The listing builds one solid part. Answer for the finished solid, in the listing's coordinates (mm). A direction names the side the tool comes from. Give positions to 0.01 mm unless a question says otherwise; leave off trailing zeros. Order: outer loops, then holes, each group sorted by start corner. A loop starts at its lowest first (then second) coordinate and runs counter-clockwise, first axis right, second up. Notation, with made-up numbers: (51.25, 13.25) -> (107.25, 13.25) arc R19 ccw to (107.25, 28.25) -> close; hole circle Ø8 at (-16, 34.5). An arc over 180 degrees is marked (long way). One line per question, with ' | ' between items. Start each with the question number.
```python
from build123d import *

# Parameters (mm, degrees)
F0_W     = 463.55
F0_H     = 158.75
F1_DEPTH = 457.2
F3_DEPTH = 158.751
F4_W     = 44.45
F4_H     = 304.8
F5_DEPTH = 381.001


with BuildPart() as f1:
    # F0 (on Top) → F1 (new body)
    with BuildSketch(Plane.XY):
        Rectangle(F0_W, F0_H)
    extrude(amount=F1_DEPTH)

    # F2 (on face) → F3 (cut, through all)
    with BuildSketch(Plane.XZ.offset(79.375)):
        Polygon((-149.225, 0), (-149.225, 304.8), (-231.775, 381), (-231.775, 0), align=None)
        Polygon((149.225, 304.8), (149.225, 0), (231.775, 0), (231.775, 381), align=None)
    extrude(amount=-F3_DEPTH, mode=Mode.SUBTRACT)

    # F4 (on face) → F5 (cut, through all)
    with BuildSketch(Plane(origin=(-149.225, 0, 0), x_dir=(0, -1, 0), z_dir=(-1, 0, 0))):
        with Locations((-57.15, 152.4)):
            Rectangle(F4_W, F4_H)
        with Locations((57.15, 152.4)):
            Rectangle(F4_W, F4_H)
    extrude(amount=-F5_DEPTH, mode=Mode.SUBTRACT)


solid = f1.part
```
(1) Consider line 1 (Y direction, x = 4, z = 241) (3 decimals); line 2 (X direction, y = -10.5, z = 38) (3 decimals); line 3 (Z direction, x = 91, y = 68). Determine where each line is inside the solid, lowest interval first.
(2) The part is cut by section D-D on y = -41.5. Determine the outline of the cut face in (x, z) (3 decimals).
(3) For faces 1 (the face through (-2, 57, 304.8)), 2 (the face through (-2, -34.925, 150)), 3 (the face through (149.225, 0, 155)), determine the directions among +Z, -Z, +X, -X, +Y, -Y from which every point of the face is accessible in a straight line to the end or side of a thin tool.
(4) The part is cut by section A-A on x = -83. Determine the outline of the cut face in (y, z) (3 decimals).
(5) Given P1, Ø13.5, axis at x = -38.5, y = 52.5, coming from the -Z side; P2, Ø1, axis at y = 19, z = 240, coming from the +X side (3 decimals); P3, Ø12, axis at x = 9.5, z = 298, coming from the -Y side (3 decimals), each flat-ended and moving along its own axis, determine where each tip first touches the part or whether it passes through.
(6) The part is cut by section C-C on z = 110. Determine the outline of the cut face in (x, y) (3 decimals), plus the area to 3 significant figures.
(7) The part is cut by section B-B on y = 10. Determine the outline of the cut face in (x, z) (3 decimals).
Result sheet:
1) line 1: y = -34.925 to 34.925 | line 2: x = -149.225 to 149.225 | line 3: z = 304.8 to 457.2
2) outline: (-231.775, 381) -> (-149.225, 304.8) -> (149.225, 304.8) -> (231.775, 381) -> (231.775, 457.2) -> (-231.775, 457.2) -> close
3) face 1: -Z, +X, -X, +Y | face 2: -Z, +X, -X, -Y | face 3: -Z, +X, +Y, -Y
4) outline: (-79.375, 304.8) -> (-34.925, 304.8) -> (-34.925, 0) -> (34.925, 0) -> (34.925, 304.8) -> (79.375, 304.8) -> (79.375, 457.2) -> (-79.375, 457.2) -> close
5) P1: stops at z = 304.8 | P2: stops at x = 149.225 | P3: stops at y = -34.925
6) outline: (-149.225, -34.925) -> (149.225, -34.925) -> (149.225, 34.925) -> (-149.225, 34.925) -> close | area: 20,800 mm^2
7) outline: (-231.775, 381) -> (-149.225, 304.8) -> (-149.225, 0) -> (149.225, 0) -> (149.225, 304.8) -> (231.775, 381) -> (231.775, 457.2) -> (-231.775, 457.2) -> close
